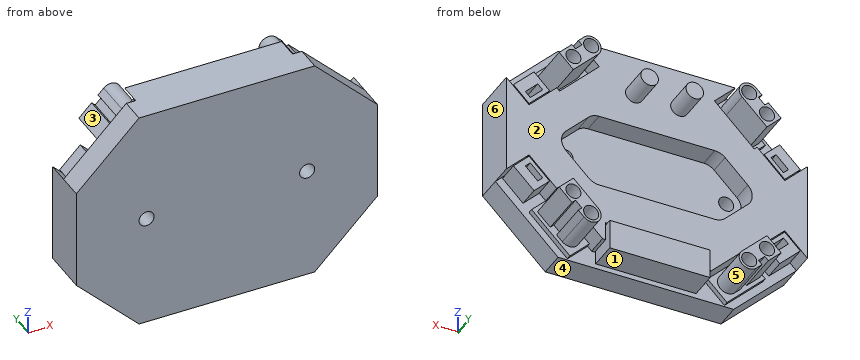
from build123d import *

# Parameters (mm, degrees)
SKETCH_1_R          = 1.5
EXTRUDE_1_DEPTH     = 5
SKETCH_2_R          = 1.5
EXTRUDE_2_DEPTH     = 9.5
CUT_EXTRUDE_1_DEPTH = 8.5
EXTRUDE_3_DEPTH     = 4.3
SKETCH_6_W          = 20
SKETCH_6_H          = 6
EXTRUDE_4_DEPTH     = 5.5
EXTRUDE_5_DEPTH     = 4.3
SKETCH_8_R          = 1.75
EXTRUDE_6_DEPTH     = 6


with BuildPart() as part:
    # 草图1 → 凸台-拉伸1 (new body)
    with BuildSketch(Plane(origin=(0, 0, 0), x_dir=(1, 0, 0), z_dir=(0, 1, 0))):
        Polygon((-30, 10), (-17.5, 22.5), (17.5, 22.5), (30, 10), (30, -10), (17.5, -22.5), (-17.5, -22.5), (-30, -10), align=None)
        with Locations(Location((-16, 0, 0), (0, 0, 270))):
            Circle(SKETCH_1_R, mode=Mode.SUBTRACT)
        with Locations(Location((16, 0, 0), (0, 0, 270))):
            Circle(SKETCH_1_R, mode=Mode.SUBTRACT)
    extrude(amount=EXTRUDE_1_DEPTH)

    # 草图2 → 凸台-拉伸2 (add)
    # profile 1 of 4: a face of its own
    with BuildSketch(Plane(origin=(0, 5, 0), x_dir=(1, 0, 0), z_dir=(0, 1, 0))):
        Polygon((-23.282485579, 14.596194078), (-19.393398282, 10.707106781), (-11.756645045, 18.343860018), (-15.645732342, 22.232947315), align=None)
        with Locations(Location((-15.751798359, 18.237794001, 0), (0, 0, 270))):
            Circle(SKETCH_2_R, mode=Mode.SUBTRACT)
        with Locations(Location((-19.287332265, 14.702260095, 0), (0, 0, 270))):
            Circle(SKETCH_2_R, mode=Mode.SUBTRACT)
    # profile 2 of 4: a face of its own
    with BuildSketch(Plane(origin=(0, 5, 0), x_dir=(1, 0, 0), z_dir=(0, 1, 0))):
        Polygon((15.645732342, 22.232947315), (11.756645045, 18.343860018), (19.393398282, 10.707106781), (23.282485579, 14.596194078), align=None)
        with Locations(Location((19.287332265, 14.702260095, 0), (0, 0, 90))):
            Circle(SKETCH_2_R, mode=Mode.SUBTRACT)
        with Locations(Location((15.751798359, 18.237794001, 0), (0, 0, 90))):
            Circle(SKETCH_2_R, mode=Mode.SUBTRACT)
    # profile 3 of 4: a face of its own
    with BuildSketch(Plane(origin=(0, 5, 0), x_dir=(1, 0, 0), z_dir=(0, 1, 0))):
        Polygon((23.282485579, -14.596194078), (19.393398282, -10.707106781), (11.756645045, -18.343860018), (15.645732342, -22.232947315), align=None)
        with Locations(Location((15.751798359, -18.237794001, 0), (0, 0, 270))):
            Circle(SKETCH_2_R, mode=Mode.SUBTRACT)
        with Locations(Location((19.287332265, -14.702260095, 0), (0, 0, 270))):
            Circle(SKETCH_2_R, mode=Mode.SUBTRACT)
    # profile 4 of 4: a face of its own
    with BuildSketch(Plane(origin=(0, 5, 0), x_dir=(1, 0, 0), z_dir=(0, 1, 0))):
        Polygon((-15.645732342, -22.232947315), (-11.756645045, -18.343860018), (-19.393398282, -10.707106781), (-23.282485579, -14.596194078), align=None)
        with Locations(Location((-19.287332265, -14.702260095, 0), (0, 0, 90))):
            Circle(SKETCH_2_R, mode=Mode.SUBTRACT)
        with Locations(Location((-15.751798359, -18.237794001, 0), (0, 0, 90))):
            Circle(SKETCH_2_R, mode=Mode.SUBTRACT)
    extrude(amount=EXTRUDE_2_DEPTH)

    # 草图3 → 切除-拉伸1 (cut)
    # profile 1 of 4: a face of its own
    with BuildSketch(Plane(origin=(0, 14.5, 0), x_dir=(1, 0, 0), z_dir=(0, 1, 0))):
        Polygon((-15.645732342, 22.232947315), (-23.282485579, 14.596194078), (-19.393398282, 10.707106781), (-11.756645045, 18.343860018), align=None)
        with BuildLine():
            Line((-14.337584797, 16.823580438), (-19.287332265, 11.87383297))
            Line((-19.287332265, 11.87383297), (-22.11575939, 14.702260095))
            Line((-22.11575939, 14.702260095), (-19.570174977, 17.247844507))
            Line((-19.570174977, 17.247844507), (-18.863068196, 16.540737726))
            Line((-18.863068196, 16.540737726), (-17.59027599, 17.813529932))
            Line((-17.59027599, 17.813529932), (-18.297382771, 18.520636713))
            Line((-18.297382771, 18.520636713), (-17.166011921, 19.652007563))
            ThreePointArc((-17.166011921, 19.652007563), (-14.337584797, 19.652007563), (-14.337584797, 16.823580438))
        make_face(mode=Mode.SUBTRACT)
    # profile 2 of 4: a face of its own
    with BuildSketch(Plane(origin=(0, 14.5, 0), x_dir=(1, 0, 0), z_dir=(0, 1, 0))):
        Polygon((11.756645045, 18.343860018), (15.645732342, 22.232947315), (23.282485579, 14.596194078), (19.393398282, 10.707106781), align=None)
        with BuildLine():
            Line((18.297382771, 18.520636713), (17.166011921, 19.652007563))
            ThreePointArc((17.166011921, 19.652007563), (14.337584797, 19.652007563), (14.337584797, 16.823580438))
            Line((14.337584797, 16.823580438), (19.287332265, 11.87383297))
            Line((19.287332265, 11.87383297), (22.11575939, 14.702260095))
            Line((22.11575939, 14.702260095), (19.570174977, 17.247844507))
            Line((19.570174977, 17.247844507), (18.863068196, 16.540737726))
            Line((18.863068196, 16.540737726), (17.59027599, 17.813529932))
            Line((17.59027599, 17.813529932), (18.297382771, 18.520636713))
        make_face(mode=Mode.SUBTRACT)
    # profile 3 of 4: a face of its own
    with BuildSketch(Plane(origin=(0, 14.5, 0), x_dir=(1, 0, 0), z_dir=(0, 1, 0))):
        Polygon((15.645732342, -22.232947315), (23.282485579, -14.596194078), (19.393398282, -10.707106781), (11.756645045, -18.343860018), align=None)
        with BuildLine():
            Line((14.337584797, -16.823580438), (19.287332265, -11.87383297))
            Line((19.287332265, -11.87383297), (22.11575939, -14.702260095))
            Line((22.11575939, -14.702260095), (19.570174977, -17.247844507))
            Line((19.570174977, -17.247844507), (18.863068196, -16.540737726))
            Line((18.863068196, -16.540737726), (17.59027599, -17.813529932))
            Line((17.59027599, -17.813529932), (18.297382771, -18.520636713))
            Line((18.297382771, -18.520636713), (17.166011921, -19.652007563))
            ThreePointArc((17.166011921, -19.652007563), (14.337584797, -19.652007563), (14.337584797, -16.823580438))
        make_face(mode=Mode.SUBTRACT)
    # profile 4 of 4: a face of its own
    with BuildSketch(Plane(origin=(0, 14.5, 0), x_dir=(1, 0, 0), z_dir=(0, 1, 0))):
        Polygon((-11.756645045, -18.343860018), (-15.645732342, -22.232947315), (-23.282485579, -14.596194078), (-19.393398282, -10.707106781), align=None)
        with BuildLine():
            Line((-18.297382771, -18.520636713), (-17.166011921, -19.652007563))
            ThreePointArc((-17.166011921, -19.652007563), (-14.337584797, -19.652007563), (-14.337584797, -16.823580438))
            Line((-14.337584797, -16.823580438), (-19.287332265, -11.87383297))
            Line((-19.287332265, -11.87383297), (-22.11575939, -14.702260095))
            Line((-22.11575939, -14.702260095), (-19.570174977, -17.247844507))
            Line((-19.570174977, -17.247844507), (-18.863068196, -16.540737726))
            Line((-18.863068196, -16.540737726), (-17.59027599, -17.813529932))
            Line((-17.59027599, -17.813529932), (-18.297382771, -18.520636713))
        make_face(mode=Mode.SUBTRACT)
    extrude(amount=-CUT_EXTRUDE_1_DEPTH, mode=Mode.SUBTRACT)

    # 草图4 → 凸台-拉伸3 (add)
    # profile 1 of 4: a face of its own
    with BuildSketch(Plane(origin=(0, 5, 0), x_dir=(1, 0, 0), z_dir=(0, 1, 0))):
        Polygon((-28.585786438, 8.86862915), (-24.484567107, 12.969848481), (-21.37329727, 9.858578644), (-25.4745166, 5.757359313), align=None)
        Polygon((-26.216978721, 8.12616703), (-23.742104986, 10.601040764), (-22.752155493, 9.61109127), (-25.227029227, 7.136217536), align=None, mode=Mode.SUBTRACT)
    # profile 2 of 4: a face of its own
    with BuildSketch(Plane(origin=(0, 5, 0), x_dir=(1, 0, 0), z_dir=(0, 1, 0))):
        Polygon((25.4745166, 5.757359313), (21.37329727, 9.858578644), (24.484567107, 12.969848481), (28.585786438, 8.86862915), align=None)
        Polygon((25.227029227, 7.136217536), (22.752155493, 9.61109127), (23.742104986, 10.601040764), (26.216978721, 8.12616703), align=None, mode=Mode.SUBTRACT)
    # profile 3 of 4: a face of its own
    with BuildSketch(Plane(origin=(0, 5, 0), x_dir=(1, 0, 0), z_dir=(0, 1, 0))):
        Polygon((28.585786438, -8.86862915), (24.484567107, -12.969848481), (21.37329727, -9.858578644), (25.4745166, -5.757359313), align=None)
        Polygon((26.216978721, -8.12616703), (23.742104986, -10.601040764), (22.752155493, -9.61109127), (25.227029227, -7.136217536), align=None, mode=Mode.SUBTRACT)
    # profile 4 of 4: a face of its own
    with BuildSketch(Plane(origin=(0, 5, 0), x_dir=(1, 0, 0), z_dir=(0, 1, 0))):
        Polygon((-25.4745166, -5.757359313), (-21.37329727, -9.858578644), (-24.484567107, -12.969848481), (-28.585786438, -8.86862915), align=None)
        Polygon((-25.227029227, -7.136217536), (-22.752155493, -9.61109127), (-23.742104986, -10.601040764), (-26.216978721, -8.12616703), align=None, mode=Mode.SUBTRACT)
    extrude(amount=EXTRUDE_3_DEPTH)

    # 草图6 → 凸台-拉伸4 (add)
    with BuildSketch(Plane(origin=(0, 5, 0), x_dir=(1, 0, 0), z_dir=(0, 1, 0))):
        with Locations((0, 18.5)):
            Rectangle(SKETCH_6_W, SKETCH_6_H)
    extrude(amount=EXTRUDE_4_DEPTH)

    # 草图5 → 凸台-拉伸5 (add)
    with BuildSketch(Plane(origin=(0, 5, 0), x_dir=(1, 0, 0), z_dir=(0, 1, 0))):
        Polygon((-30, 10), (-30, -10), (-25.4745166, -5.4745166), (-19.959083707, -10.989949494), (-19.393398282, -10.424264069), (-11.473802333, -18.343860018), (-15.629942315, -22.5), (15.629942315, -22.5), (11.473802333, -18.343860018), (19.393398282, -10.424264069), (19.959083707, -10.989949494), (25.4745166, -5.4745166), (30, -10), (30, 10), (25.4745166, 5.4745166), (19.959083707, 10.989949494), (19.393398282, 10.424264069), (10.817662351, 19), (10.2, 19), (10.2, 15.3), (-10.2, 15.3), (-10.2, 19), (-10.817662351, 19), (-19.393398282, 10.424264069), (-19.959083707, 10.989949494), (-25.4745166, 5.4745166), align=None)
        with BuildLine():
            Line((-18.121320344, 2.121320344), (-13.604055577, 6.63858511))
            ThreePointArc((-13.604055577, 6.63858511), (-12.649908859, 7.276125564), (-11.524416066, 7.5))
            Line((-11.524416066, 7.5), (11.524416066, 7.5))
            ThreePointArc((11.524416066, 7.5), (12.649908859, 7.276125564), (13.604055577, 6.63858511))
            Line((13.604055577, 6.63858511), (18.121320344, 2.121320344))
            ThreePointArc((18.121320344, 2.121320344), (19, 0), (18.121320344, -2.121320344))
            Line((18.121320344, -2.121320344), (13.604055577, -6.63858511))
            ThreePointArc((13.604055577, -6.63858511), (12.649908859, -7.276125564), (11.524416066, -7.5))
            Line((11.524416066, -7.5), (-11.524416066, -7.5))
            ThreePointArc((-11.524416066, -7.5), (-12.649908859, -7.276125564), (-13.604055577, -6.63858511))
            Line((-13.604055577, -6.63858511), (-18.121320344, -2.121320344))
            ThreePointArc((-18.121320344, -2.121320344), (-19, 0), (-18.121320344, 2.121320344))
        make_face(mode=Mode.SUBTRACT)
    extrude(amount=EXTRUDE_5_DEPTH)

    # 草图8 → 凸台-拉伸6 (add)
    with BuildSketch(Plane(origin=(0, 9.3, 0), x_dir=(1, 0, 0), z_dir=(0, 1, 0))):
        with Locations(Location((-4.5, -14.5, 0), (0, 0, 270))):
            Circle(SKETCH_8_R)
        with Locations(Location((4.5, -14.5, 0), (0, 0, 270))):
            Circle(SKETCH_8_R)
    extrude(amount=EXTRUDE_6_DEPTH)


solid = part.part
Source: CAD feature listing. Evaluate the final solid. Frame: model axes, mm. Face numbers are marked on the shaded views. A direction names the side the tool comes from. Coordinates: 2 decimals unless noted, no trailing zeros. Order: outer loops, then holes, each group sorted by start corner. A loop starts at its lowest first (then second) coordinate and runs counter-clockwise, first axis right, second up.
Item 1: First-contact query: P1, Ø1, axis at x = 24.5, z = -9.5, coming from the +Y side; P2, Ø3, axis at y = 7.5, z = -17, coming from the +X side; P3, Ø3, axis at x = 15, z = -14.5, coming from the +Y side; P4, Ø5, axis at y = 13, z = -7, coming from the +X side. Flat tips, straight axial feed; report the tip coordinate or a pass-through.
Output values:
P1: stops at y = 9.3
P2: stops at x = 21.32
P3: stops at y = 14.5
P4: passes through
Item 2: Cut plane A-A (z = 0). Return loops of the section in (x, y).
Output values:
outline: (-30, 0) - (-17.5, 0) - (-17.5, 5) - (-19, 5) - (-19, 9.3) - (-30, 9.3) - close; (-14.5, 0) - (14.5, 0) - (14.5, 5) - (-14.5, 5) - close; (17.5, 0) - (30, 0) - (30, 9.3) - (19, 9.3) - (19, 5) - (17.5, 5) - close
Item 3: Pull-direction query (Z, two-part tool) for the marked faces 4, 5 and 6; classes: pulls with the +Z half, pulls with the -Z half, needs draft (parallel to the pull), parting line crosses it, or undercut.
Output values:
face 4: pulls with the -Z half
face 5: undercut
face 6: needs draft
Item 4: Set-up query: the marked faces 1, 2 and 3. Return all of +Z, -Z, +X, -X, +Y, -Y with unobstructed straight access to the full face (end or side cutting, diameter ignored); none if empty.
Output values:
face 1: -Z, +Y
face 2: +Y
face 3: +Z, -X, +Y
Item 5: Cut plane B-B (x = 4.5). Return loops of the section in (y, z), plus the area to 3 significant figures.
Output values:
outline: (0, -22.5) - (5, -22.5) - (5, -21.5) - (10.5, -21.5) - (10.5, -15.5) - (5, -15.5) - (5, -15.3) - (9.3, -15.3) - (9.3, -7.5) - (5, -7.5) - (5, 7.5) - (9.3, 7.5) - (9.3, 12.75) - (15.3, 12.75) - (15.3, 16.25) - (9.3, 16.25) - (9.3, 22.5) - (0, 22.5) - close
area: 377 mm2
Item 6: Cut plane C-C (y = 11.5). Count the separate pieces of the cut face and the enclosed holes in it, plus the area to 3 significant figures.
Output values:
separate pieces: 6
enclosed holes: 8
area: 92.6 mm2
Item 7: Material intervals for line 1 (Z direction, x = 4.5, y = 8.25); line 2 (X direction, y = 1, z = 0); line 3 (Z direction, x = 13.5, y = 7), sorted ascending.
Output values:
line 1: z = -21.5 to -15.5, -15.3 to -7.5, 7.5 to 22.5
line 2: x = -30 to -17.5, -14.5 to 14.5, 17.5 to 30
line 3: z = -16.32 to -6.74, 6.74 to 16.32, 20.37 to 22.5
